Source: CAD feature listing. Evaluate the final solid. Frame: model axes, mm. A direction names the side the tool comes from. Coordinates: 2 decimals unless noted, no trailing zeros. Loops run counter-clockwise (first coordinate to the right, second up) from the corner with the lowest first, then second, coordinate; pieces in that order, holes last. Notation, with made-up numbers: M 32,54 L 42,54 A28 cw 42,87 Z; hole C -20,-14 d3. An arc over 180 degrees is marked long. Write each question's results on one line, items separated by ' | '. Start each with the question number.
from build123d import *

# Parameters (mm, degrees)
SKETCH1_W               = 10
SKETCH1_H               = 70
BOSS_EXTRUDE1_DEPTH     = 3
SKETCH2_W               = 3
SKETCH2_H               = 70
BOSS_EXTRUDE2_DEPTH     = 10
SKETCH3_R               = 1.35
CUT_EXTRUDE1_DEPTH      = 1
CUT_EXTRUDE1_DEPTH_BACK = 14
SKETCH4_R               = 1.35
CUT_EXTRUDE2_DEPTH      = 10
CHAMFER1_SIZE           = 10
CHAMFER1_SIZE2          = 5.773502692
CHAMFER1_PART_2_SIZE    = 10
CHAMFER1_PART_2_SIZE2   = 5.773502692
SKETCH5_W               = 3
SKETCH5_H               = 54
CUT_EXTRUDE3_DEPTH      = 10


with BuildPart() as part:
    # Sketch1 → Boss-Extrude1 (new body)
    with BuildSketch(Plane(origin=(0, 0, 0), x_dir=(1, 0, 0), z_dir=(0, 1, 0))):
        with Locations((5, 0)):
            Rectangle(SKETCH1_W, SKETCH1_H)
    extrude(amount=BOSS_EXTRUDE1_DEPTH)

    # Sketch2 → Boss-Extrude2 (add)
    with BuildSketch(Plane.XZ):
        with Locations((1.5, 0)):
            Rectangle(SKETCH2_W, SKETCH2_H)
    extrude(amount=BOSS_EXTRUDE2_DEPTH)

    # Sketch3 → Cut-Extrude1 (cut, two sides)
    with BuildSketch(Plane(origin=(0, 3, 0), x_dir=(1, 0, 0), z_dir=(0, 1, 0))) as cut_extrude1_sk:
        with Locations((5, 31)):
            Circle(SKETCH3_R)
        with Locations((5, -31)):
            Circle(SKETCH3_R)
    extrude(amount=CUT_EXTRUDE1_DEPTH, mode=Mode.SUBTRACT)
    extrude(cut_extrude1_sk.sketch, amount=-CUT_EXTRUDE1_DEPTH_BACK, mode=Mode.SUBTRACT)

    # Sketch4 → Cut-Extrude2 (cut)
    with BuildSketch(Plane(origin=(3, 0, 0), x_dir=(0, 0, -1), z_dir=(1, 0, 0))):
        with Locations((25, -5)):
            Circle(SKETCH4_R)
        with Locations((-25, -5)):
            Circle(SKETCH4_R)
    extrude(amount=-CUT_EXTRUDE2_DEPTH, mode=Mode.SUBTRACT)

    # Chamfer1
    chamfer1_edges = [part.edges().sort_by_distance(p)[0] for p in [
        (1.5, -10, -35),
    ]]
    chamfer1_side = [part.faces().sort_by_distance(p)[0] for p in [
        (9.835987805, 1.5, -35),
    ]]
    chamfer(chamfer1_edges, length=CHAMFER1_SIZE, length2=CHAMFER1_SIZE2, reference=chamfer1_side[0])

    # Chamfer1 part 2
    chamfer1_part_2_edges = [part.edges().sort_by_distance(p)[0] for p in [
        (1.5, -10, 35),
    ]]
    chamfer1_part_2_side = [part.faces().sort_by_distance(p)[0] for p in [
        (0.164012195, -3.5, 35),
    ]]
    chamfer(chamfer1_part_2_edges, length=CHAMFER1_PART_2_SIZE, length2=CHAMFER1_PART_2_SIZE2, reference=chamfer1_part_2_side[0])

    # Sketch5 → Cut-Extrude3 (cut)
    with BuildSketch(Plane(origin=(0, 3, 0), x_dir=(1, 0, 0), z_dir=(0, 1, 0))):
        with Locations((8.5, 0)):
            Rectangle(SKETCH5_W, SKETCH5_H)
    extrude(amount=-CUT_EXTRUDE3_DEPTH, mode=Mode.SUBTRACT)


solid = part.part
Item 1: Access query for faces 4 (the flat face through (3, -5, 0)), 5 (the flat face through (10, 1, 31)), 6 (the flat face through (8, 2, -27)). Directions: +Z, -Z, +X, -X, +Y, -Y. A direction counts if a zero-diameter tool reaches every point of the face in a straight line with its end or side. Return the directions, or none.
Item 2: First-contact query: pin 1 Ø5 at (y, z) = (-4.5, 12) entering from +X; pin 2 Ø2.5 at (y, z) = (1, -12) entering from +X; pin 3 Ø5 at (x, z) = (9, 5) entering from -Y. Flat tips, straight axial feed; report the tip coordinate or a pass-through.
Item 3: Line query: probe 1 along Z at (x, y) = (5, 1.5); probe 2 along X at (y, z) = (0.75, -31); probe 3 along Y at (x, z) = (0.85, -25). Output: solid intervals per line, ascending.
Item 4: Mould query, pull axis Y, two halves, no side actions, for faces 1 (the flat face through (8, 2, 27)), 2 (the cylindrical face through (1.521, -4.594, -26.288)), 3 (the flat face through (4, 3, 0)). Classes: +Y half, -Y half, draft (parallel to the pull), parting line (faces both ways), or undercut.
Item 5: Cut plane C-C (y = -5). Output: boundary loops of the cut face in (x, z), then the cut area to 3 significant figures.
Item 6: Cut plane D-D (x = 1). Output: boundary loops of the cut face in (y, z).
Item 7: Cut plane B-B (x = 5). Output: boundary loops of the cut face in (y, z).
Item 8: Cut plane A-A (x = 8.75). Output: boundary loops of the cut face in (y, z).
Response values:
1) face 4: +Z, -Z, +X, -Y | face 5: +Z, -Z, +X, +Y, -Y | face 6: +X, +Y, -Y
2) pin 1: stops at x = 3 | pin 2: stops at x = 7 | pin 3: stops at y = 0
3) probe 1: z = -35 to -32.35, -29.65 to 29.65, 32.35 to 35 | probe 2: x = 0 to 3.65, 6.35 to 10 | probe 3: y = -10 to -6.35, -3.65 to 3
4) face 1: draft | face 2: undercut | face 3: +Y half
5) outline: M 0,-32.11 L 3,-32.11 L 3,-26.35 L 0,-26.35 Z; M 0,-23.65 L 3,-23.65 L 3,23.65 L 0,23.65 Z; M 0,26.35 L 3,26.35 L 3,32.11 L 0,32.11 Z | area: 176 mm2
6) outline: M -10,-29.23 L 0,-35 L 3,-35 L 3,35 L 0,35 L -10,29.23 Z; hole C -5,-25 d2.7; hole C -5,25 d2.7
7) outline: M 0,-35 L 3,-35 L 3,-32.35 L 0,-32.35 Z; M 0,-29.65 L 3,-29.65 L 3,29.65 L 0,29.65 Z; M 0,32.35 L 3,32.35 L 3,35 L 0,35 Z
8) outline: M 0,-35 L 3,-35 L 3,-27 L 0,-27 Z; M 0,27 L 3,27 L 3,35 L 0,35 Z
